from build123d import *

# Parameters (mm, degrees)
SKETCH_W     = 50.5
SKETCH_H     = 17
PAD_DEPTH    = 9
SKETCH001_W  = 2.6
SKETCH001_H  = 29
PAD001_DEPTH = 25.25
SKETCH002_W  = 31
SKETCH002_H  = 2.6
PAD002_DEPTH = 2.6


with BuildPart() as part:
    # Sketch → Pad (new body)
    with BuildSketch(Plane.XY):
        Rectangle(SKETCH_W, SKETCH_H)
    extrude(amount=PAD_DEPTH)

    # Sketch001 → Pad001 (join, symmetric)
    with BuildSketch(Plane.YZ):
        with Locations((7.2, 14.5)):
            Rectangle(SKETCH001_W, SKETCH001_H)
    extrude(amount=PAD001_DEPTH, both=True)

    # Sketch002 (on Face5 of Pad001) → Pad002 (join)
    with BuildSketch(Plane(origin=(0, 8.5, 0), x_dir=(-1, 0, 0), z_dir=(0, 1, 0))):
        with Locations((0, 27.7)):
            Rectangle(SKETCH002_W, SKETCH002_H)
    extrude(amount=PAD002_DEPTH)


solid = part.part
Read the model definition and answer for the solid it produces. Units are mm, in the model's axes. A direction names the side the tool comes from. Coordinates: 2 decimals unless noted, no trailing zeros. Loops run counter-clockwise (first coordinate to the right, second up) from the corner with the lowest first, then second, coordinate; pieces in that order, holes last. Notation, with made-up numbers: (-23.75, 78.25) -> (30.25, 78.25) arc R27 cw to (30.25, 97.25) -> close; hole circle Ø1 at (55.25, 48.5). An arc over 180 degrees is marked (long way). Answer in a Markdown table with one row per item.
Item 1: A cutting plane is placed at C-C on y = 3.25. Determine the outline of the cut face in (x, z).
Returned:
| item | result |
|---|---|
| outline | (-25.25, 0) -> (25.25, 0) -> (25.25, 9) -> (-25.25, 9) -> close |
Item 2: Straight lines are drawn through the part: line 1 along Z through (x, y) = (-15.5, -7.25); line 2 along Y through (x, z) = (-15, 3.25); line 3 along Y through (x, z) = (21, 22.25). For each, find the intervals that lie inside material, in ascending order. Write a range as [from, to].
Returned:
| item | result |
|---|---|
| line 1 | z = [0, 9] |
| line 2 | y = [-8.5, 8.5] |
| line 3 | y = [5.9, 8.5] |
Item 3: For faces 1 (the flat face through (15.5, 10, 28)), 2 (the flat face through (0, 10, 26.4)), 3 (the flat face through (0, 8, 29)), 4 (the flat face through (0, -1, 9)), 5 (the flat face through (-15.5, 10, 28)), determine the directions among +Z, -Z, +X, -X, +Y, -Y from which every point of the face is accessible in a straight line to the end or side of a thin tool.
Returned:
| item | result |
|---|---|
| face 1 | +Z, -Z, +X, +Y |
| face 2 | -Z, +X, -X, +Y |
| face 3 | +Z, +X, -X, +Y, -Y |
| face 4 | +Z, +X, -X, -Y |
| face 5 | +Z, -Z, -X, +Y |
Item 4: A cutting plane is placed at D-D on x = -9. Determine the outline of the cut face in (y, z).
Returned:
| item | result |
|---|---|
| outline | (-8.5, 0) -> (8.5, 0) -> (8.5, 26.4) -> (11.1, 26.4) -> (11.1, 29) -> (5.9, 29) -> (5.9, 9) -> (-8.5, 9) -> close |
Item 5: A cutting plane is placed at A-A on z = 27. Determine the outline of the cut face in (x, y).
Returned:
| item | result |
|---|---|
| outline | (-25.25, 5.9) -> (25.25, 5.9) -> (25.25, 8.5) -> (15.5, 8.5) -> (15.5, 11.1) -> (-15.5, 11.1) -> (-15.5, 8.5) -> (-25.25, 8.5) -> close |
Item 6: Each of these flat-tipped pins is pushed along its axis until it touches: P1, Ø8, axis at x = -4.5, y = 3.5, coming from the +Z side; P2, Ø3, axis at x = 6.5, y = -1, coming from the +Z side; P3, Ø2, axis at y = 10.5, z = 28, coming from the -X side; P4, Ø1.3, axis at y = 10.5, z = 27, coming from the +X side. Where does it stop, or does it pass through?
Returned:
| item | result |
|---|---|
| P1 | stops at z = 29 |
| P2 | stops at z = 9 |
| P3 | stops at x = -15.5 |
| P4 | stops at x = 15.5 |
Item 7: A cutting plane is placed at B-B on x = -17.5. Determine the outline of the cut face in (y, z), plus the area to 3 significant figures.
Returned:
| item | result |
|---|---|
| outline | (-8.5, 0) -> (8.5, 0) -> (8.5, 29) -> (5.9, 29) -> (5.9, 9) -> (-8.5, 9) -> close |
| area | 205 mm^2 |
